from build123d import *

# Parameters (mm, degrees)
SK_REARHOLE_R           = 1.25
REAR_TAPPED_HOLE_DEPTH  = 8
REAR_HOLE_PATTERN_COUNT = 6
SK_CONNECTOR_W          = 18
SK_CONNECTOR_H          = 12
CONNECTOR_ZONE_DEPTH    = 14


with BuildPart() as part:
    # SK_Body → Housing_Body (revolve)
    with BuildSketch(Plane(origin=(0, 0, 0), x_dir=(1, 0, 0), z_dir=(0, 1, 0))):
        Polygon((0, 0), (36.25, 0), (39.25, 3), (39.25, 40.5), (36.25, 40.5), (0, 40.5), align=None)
    revolve(axis=Axis((0, 0, 10), (0, 0, -1)))

    # SK_RearHole → Rear_Tapped_Hole (cut)
    with BuildSketch(Plane.XY.offset(-40.5)):
        with Locations((33, 0)):
            Circle(SK_REARHOLE_R)
    rear_tapped_hole = extrude(amount=REAR_TAPPED_HOLE_DEPTH, mode=Mode.SUBTRACT)

    # Rear_Hole_Pattern: Rear_Tapped_Hole ×6 about axis
    rear_hole_pattern_axis = Axis((0, 0, 0), (0, 0, 1))
    for i in range(1, REAR_HOLE_PATTERN_COUNT):
        add(rear_tapped_hole.rotate(rear_hole_pattern_axis, i * 360 / REAR_HOLE_PATTERN_COUNT), mode=Mode.SUBTRACT)

    # SK_Connector → Connector_Zone (add)
    with BuildSketch(Plane.XY.offset(-40.5)):
        with Locations((0, 41.25)):
            Rectangle(SK_CONNECTOR_W, SK_CONNECTOR_H)
    extrude(amount=CONNECTOR_ZONE_DEPTH)


solid = part.part
For this review, take the finished solid that the model builds, in its own axes (mm). A direction names the side the tool comes from. Give positions to 0.01 mm unless a question says otherwise; leave off trailing zeros. Order: outer loops, then holes, each group sorted by start corner. A loop starts at its lowest first (then second) coordinate and runs counter-clockwise, first axis right, second up. Notation, with made-up numbers: (-39, 14) - (-9, 14) arc R30 cw to (-9, 43) - close; hole circle Ø2 at (76, 78.5). An arc over 180 degrees is marked (long way). Answer as a JSON object with one key per item and string values. Group by question number.
Item 1: Clearance check with flat-ended pins moving along their axes: pin 1 Ø1.5 at (y, z) = (37, -15.5) entering from +X; pin 2 Ø10 at (y, z) = (36, -23) entering from -X; pin 3 Ø7 at (y, z) = (42.5, -36) entering from -X. State where each tip first meets the part, or that it passes through.
Item 2: Machinability: for faces 4 (the flat face through (-9, 43, -34)), 5 (the flat face through (17, -29, -32.5)), 6 (the conical face through (-7.899, 35.571, -0.188)), which of the approach directions +Z, -Z, +X, -X, +Y, -Y give a long, thin tool a straight path to every point of the face, cutting with its end or side? Answer none if there is none.
Item 3: Take a section at C-C on z = -24.5. Give the boundary of the cut face in (x, y).
Item 4: Wall thickness on line 1 along Y through (x, z) = (16.5, -36.75); line 2 along Y through (x, z) = (26, -1.5); line 3 along Y through (x, z) = (-33, -36.75): over which ranges is each line inside the solid? List them lowest first.
Item 5: Take a section at B-B on z = -36. Give the boundary of the cut face in (x, y) (3 decimals), and give its area (3 significant figures).
Item 6: Take a section at D-D on z = -31.5. Give the boundary of the cut face in (x, y), and give its area (3 significant figures).
Item 7: Take a section at A-A on y = 0. Give the boundary of the cut face in (x, z).
Item 8: Draft analysis for pull direction Y (two halves, no side actions). For faces 1 (the flat face through (-1, 3, -40.5)), 2 (the flat face through (-17, 29, -32.5)), 3 (the flat face through (0, 47.25, -34)), state which applies: pulls with the +Y half, pulls with the -Y half, needs draft (parallel to the pull), parting line crosses it, or undercut.
Reported:
{
 "1": {"pin 1": "x = 15.05", "pin 2": "x = -24.07", "pin 3": "x = -9"},
 "2": {"face 4": "+Z, -Z, -X, +Y", "face 5": "-Z", "face 6": "+Z"},
 "3": {"outline": "circle Ø78.5 at (0, 0)"},
 "4": {"line 1": "-35.61 to -29.83, -27.33 to 27.33, 29.83 to 35.61", "line 2": "-27.37 to 27.37", "line 3": "-21.25 to -1.25, 1.25 to 21.25"},
 "5": {"outline": "(-9, 38.204) arc R39.25 ccw (long way) to (9, 38.204) - (9, 47.25) - (-9, 47.25) - close; hole circle Ø2.5 at (-33, 0); hole circle Ø2.5 at (-16.5, -28.579); hole circle Ø2.5 at (-16.5, 28.579); hole circle Ø2.5 at (16.5, -28.579); hole circle Ø2.5 at (16.5, 28.579); hole circle Ø2.5 at (33, 0)", "area": "4,960 mm^2"},
 "6": {"outline": "(-9, 38.2) arc R39.25 ccw (long way) to (9, 38.2) - (9, 47.25) - (-9, 47.25) - close", "area": "4,990 mm^2"},
 "7": {"outline": "(-39.25, -40.5) - (-34.25, -40.5) - (-34.25, -32.5) - (-31.75, -32.5) - (-31.75, -40.5) - (31.75, -40.5) - (31.75, -32.5) - (34.25, -32.5) - (34.25, -40.5) - (39.25, -40.5) - (39.25, -3) - (36.25, 0) - (-36.25, 0) - (-39.25, -3) - close"},
 "8": {"face 1": "needs draft", "face 2": "undercut", "face 3": "pulls with the +Y half"}
}
